Check sheet for the drawn part. Datum: minimum x, y, z corner. Units: mm. A direction names the side the tool comes from. Give positions to 0.01 mm unless a question says otherwise; leave off trailing zeros. Order: outer loops, then holes, each group sorted by start corner. A loop starts at its lowest first (then second) coordinate and runs counter-clockwise, first axis right, second up. Notation, with made-up numbers: M 20,87 L 75,87 A33 cw 75,126 Z; hole C 48.5,-38.75 d2. An arc over 180 degrees is marked long. Answer as CSV lines item,"result". Start each with the question number.
Q1. Section check C-C, the plane x = 30. Record the boundary of the cut face in (y, z), then the cut area to 3 significant figures.
Q2. Mould release check, pull along Y, two halves, no side actions. Record for the marked faces 6, 7 and 8: +Y half, -Y half, draft (parallel to the pull), parting line (faces both ways), or undercut.
Q3. Go/stop test with flat-tipped pins: pin 1 (7.5 mm diameter, centred on x = 18.5, z = 24.5, fed in from +Y); pin 2 (5 mm diameter, centred on y = 7, z = 5, fed in from +X); pin 3 (2 mm diameter, centred on x = 32, y = 1.5, fed in from -Z). Record where each tip stops, or that it passes through.
Q4. Section check B-B, the plane z = 21.5. Record the boundary of the cut face in (x, y).
Q5. Thickness scan on line 1 (Y direction, x = 17, z = 5); line 2 (Y direction, x = 5.5, z = 32); line 3 (Z direction, x = 3, y = 2.75). Record the ranges inside material, lowest first.
Q6. Set-up check for the marked faces 1, 2, 3, 4 and 5: record each of +Z, -Z, +X, -X, +Y, -Y from which the full face is reachable in a straight line by a thin tool's end or side.
Q7. Section check A-A, the plane x = 15.5. Record the boundary of the cut face in (y, z).
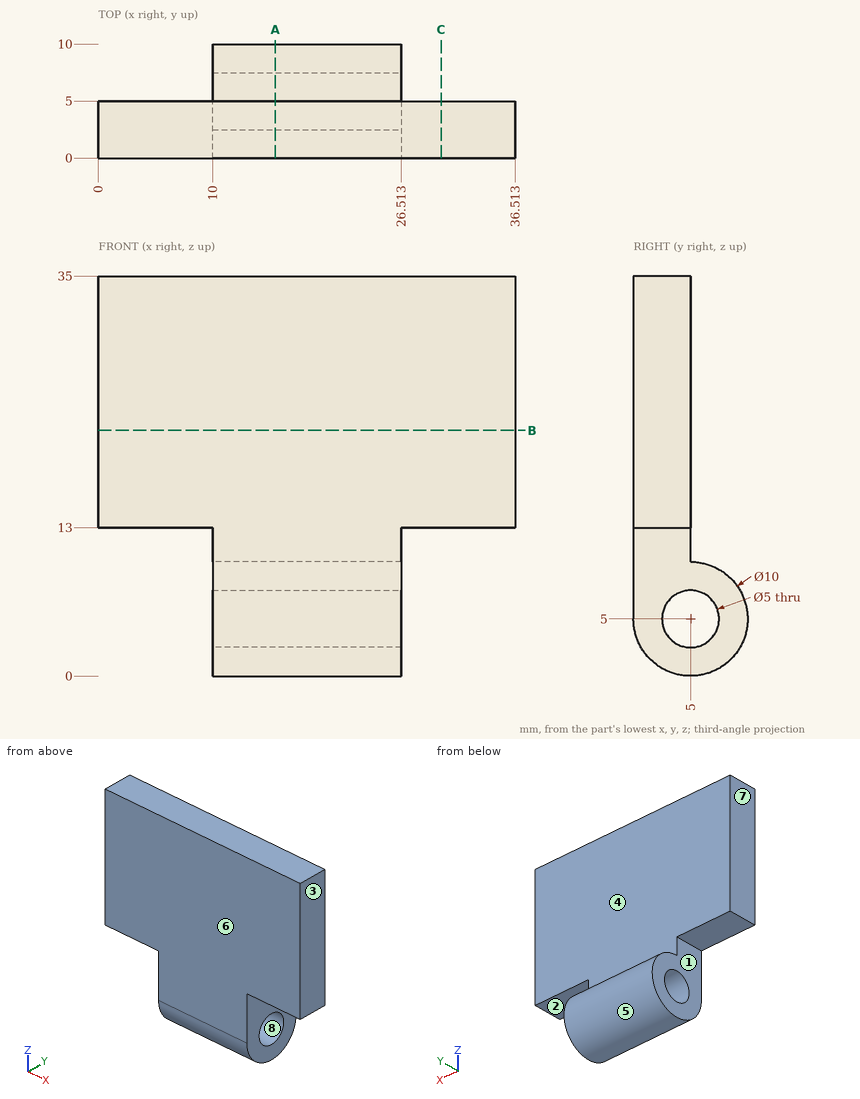
Answer block:
1,outline,"M 0,13 L 5,13 L 5,35 L 0,35 Z"
1,area,"110 mm2"
2,face 6,"-Y half"
2,face 7,"draft"
2,face 8,"undercut"
3,pin 1,"stops at y = 5"
3,pin 2,"stops at x = 26.51"
3,pin 3,"stops at z = 13"
4,outline,"M 0,0 L 36.51,0 L 36.51,5 L 0,5 Z"
5,line 1,"y = 0 to 2.5, 7.5 to 10"
5,line 2,"y = 0 to 5"
5,line 3,"z = 13 to 35"
6,face 1,"-Z, -X, +Y, -Y"
6,face 2,"-Z, +X, +Y, -Y"
6,face 3,"+Z, -Z, +X, +Y, -Y"
6,face 4,"+Z, +X, -X, +Y"
6,face 5,"+X, -X"
7,outline,"M 0,5 A5 ccw long 5,10 L 5,35 L 0,35 Z; hole C 5,5 d5"
